Source: CAD feature listing. Evaluate the final solid. Frame: model axes, mm. A direction names the side the tool comes from. Round coordinates to 2 decimals unless told otherwise and drop trailing zeros. Order: outer loops, then holes, each group sorted by start corner. A loop starts at its lowest first (then second) coordinate and runs counter-clockwise, first axis right, second up. Notation, with made-up numbers: (-1, 56.25) - (24, 56.25) arc R13 cw to (24, 76.25) - close; hole circle Ø6 at (80.25, 34.25). An arc over 180 degrees is marked (long way). Return JSON: item names as keys, results as strings. Group by question number.
1) Section C-C, the plane z = 3.5. Return loops of the section in (x, y), plus the area to 3 significant figures.
2) Section D-D, the plane y = 103. Return loops of the section in (x, z), plus the area to 3 significant figures.
3) Section B-B, the plane x = 434.5. Return loops of the section in (y, z).
4) Section A-A, the plane y = 183.5. Return loops of the section in (x, z), plus the area to 3 significant figures.
5) Access query for faces 1 (the flat face through (-500, 99, 5)), 2 (the flat face through (-490, 99, 5)). Directions: +Z, -Z, +X, -X, +Y, -Y. A direction counts if a zero-diameter tool reaches every point of the face in a straight line with its end or side. Return the directions, or none.
6) Ray query, line 1 (Z direction, x = -380.5, y = 162.5); line 2 (X direction, y = 100.5, z = -122.5); line 3 (Z direction, x = 412.5, y = 13.5). Return the intervals inside material, ascending. Write a range as from..to.
7) Contact query for a flat-ended pin moving along its axis: P1, Ø5, axis at x = 386, z = 344.5, coming from the -Y side. Output: stop coordinate, or through.
8) Mould query, pull axis Z, two halves, no side actions, for faces 3 (the flat face through (500, 99, 5)), 4 (the flat face through (-7, 99, -350)), 5 (the flat face through (-7, 99, -340)). Classes: pulls with the +Z half, pulls with the -Z half, needs draft (parallel to the pull), parting line crosses it, or undercut.
```python
from build123d import *

# Parameters (mm, degrees)
SKETCH1_W           = 1000
SKETCH1_H           = 700
SKETCH1_W_2         = 980
SKETCH1_H_2         = 680
BOSS_EXTRUDE1_DEPTH = 200
SKETCH2_W           = 100
SKETCH2_H           = 160
CUT_EXTRUDE1_DEPTH  = 200


with BuildPart() as part:
    # Sketch1 → Boss-Extrude1 (new body)
    with BuildSketch(Plane(origin=(0, 0, 0), x_dir=(1, 0, 0), z_dir=(0, 1, 0))):
        Rectangle(SKETCH1_W, SKETCH1_H)
        Rectangle(SKETCH1_W_2, SKETCH1_H_2, mode=Mode.SUBTRACT)
    extrude(amount=BOSS_EXTRUDE1_DEPTH)

    # Sketch2 → Cut-Extrude1 (cut)
    with BuildSketch(Plane.XY.offset(350)):
        with Locations((400, 80)):
            Rectangle(SKETCH2_W, SKETCH2_H)
    extrude(amount=-CUT_EXTRUDE1_DEPTH, mode=Mode.SUBTRACT)


solid = part.part
```
Geometry check:
{
 "1": {"outline": "(-500, 0) - (-490, 0) - (-490, 200) - (-500, 200) - close; (490, 0) - (500, 0) - (500, 200) - (490, 200) - close", "area": "4,000 mm2"},
 "2": {"outline": "(-500, -350) - (500, -350) - (500, 350) - (450, 350) - (450, 340) - (490, 340) - (490, -340) - (-490, -340) - (-490, 340) - (350, 340) - (350, 350) - (-500, 350) - close", "area": "32,600 mm2"},
 "3": {"outline": "(0, -350) - (200, -350) - (200, -340) - (0, -340) - close; (160, 340) - (200, 340) - (200, 350) - (160, 350) - close"},
 "4": {"outline": "(-500, -350) - (500, -350) - (500, 350) - (-500, 350) - close; hole (-490, -340) - (490, -340) - (490, 340) - (-490, 340) - close", "area": "33,600 mm2"},
 "5": {"face 1": "+Z, -Z, -X, +Y, -Y", "face 2": "+Y, -Y"},
 "6": {"line 1": "-350..-340, 340..350", "line 2": "-500..-490, 490..500", "line 3": "-350..-340"},
 "7": {"P1": "y = 160"},
 "8": {"face 3": "needs draft", "face 4": "pulls with the -Z half", "face 5": "undercut"}
}
